```python
from build123d import *

# Parameters (mm, degrees)
F0_R     = 30
F0_R_2   = 17.5
F1_DEPTH = 20
F2_R     = 100
F3_DEPTH = 20.001


with BuildPart() as f1:
    # F0 (on Front) → F1 (new body)
    with BuildSketch(Plane.XZ):
        Circle(F0_R)
        Circle(F0_R_2, mode=Mode.SUBTRACT)
    extrude(amount=-F1_DEPTH)

    # F2 (on face) → F3 (cut, through all)
    with BuildSketch(Plane.XZ):
        Circle(F2_R)
        with BuildLine():
            ThreePointArc((29.9421970705, 1.8614066163), (29.9855457856, 0.9311519438), (30, 0))
            ThreePointArc((30, 0), (25.5026684247, -15.7991741309), (13.3590731187, -26.8614066163))
            Line((13.3590731187, -26.8614066163), (0, -50))
            Line((0, -50), (-13.3590731187, -26.8614066163))
            ThreePointArc((-13.3590731187, -26.8614066163), (-25.9807621135, -15), (-29.9421970705, 1.8614066163))
            Line((-29.9421970705, 1.8614066163), (-43.3012701892, 25))
            Line((-43.3012701892, 25), (-16.5831239518, 25))
            ThreePointArc((-16.5831239518, 25), (0, 30), (16.5831239518, 25))
            Line((16.5831239518, 25), (43.3012701892, 25))
            Line((43.3012701892, 25), (29.9421970705, 1.8614066163))
        make_face(mode=Mode.SUBTRACT)
        with BuildLine():
            Line((-16.5831239518, 25), (16.5831239518, 25))
            ThreePointArc((16.5831239518, 25), (0, 30), (-16.5831239518, 25))
        make_face()
        with BuildLine():
            ThreePointArc((-29.9421970705, 1.8614066163), (-25.9807621135, -15), (-13.3590731187, -26.8614066163))
            Line((-13.3590731187, -26.8614066163), (-29.9421970705, 1.8614066163))
        make_face()
        with BuildLine():
            ThreePointArc((13.3590731187, -26.8614066163), (25.5026684247, -15.7991741309), (30, 0))
            ThreePointArc((30, 0), (29.9855457856, 0.9311519438), (29.9421970705, 1.8614066163))
            Line((29.9421970705, 1.8614066163), (13.3590731187, -26.8614066163))
        make_face()
    extrude(amount=-F3_DEPTH, mode=Mode.SUBTRACT)


solid = f1.part
```
Design review of the part built by this model. Coordinates are the model's own, in mm. Round coordinates to 2 decimals unless told otherwise and drop trailing zeros. Write each loop counter-clockwise with the first axis right and the second up, starting at its lowest first coordinate (ties: lowest second). Pieces come first, ordered by that corner, then holes. Notation, with made-up numbers: (8.25, 35.25) -> (28.25, 35.25) arc R14 cw to (28.25, 43.25) -> close; hole circle Ø3 at (88, 41.5). An arc over 180 degrees is marked (long way). Write item = value, one per line. Start each with the question number.
1) Clearance check with flat-ended pins moving along their axes: pin 1 (12 mm diameter, centred on x = -14.5, z = -5.5, fed in from -Y); pin 2 (6 mm diameter, centred on x = 12.5, y = 15, fed in from -Z); pin 3 (1 mm diameter, centred on y = 5.5, z = -3, fed in from +X); pin 4 (3 mm diameter, centred on x = -3.5, y = 15.5, fed in from -Z). State where each tip first meets the part, or that it passes through.
2) Take a section at B-B, the plane y = 7.75. State the section outline as (x, z) points.
3) Take a section at A-A, the plane x = 0. State the section outline as (y, z) points.
4) Wall thickness on probe 1 along Z at (x, y) = (0, 7.25); probe 2 along X at (y, z) = (14, 16); probe 3 along Z at (x, y) = (-11.5, 13.25): over which ranges is each line inside the solid? List them lowest first. Write a range as from..to.
5) Take a section at C-C, the plane z = 0. State the section outline as (x, y) points, plus the area to 3 significant figures.
6) Mouldability with a two-part tool opening along Z and no side actions: class faces 1 (the face through (-21.535, 9.86, -12.701)), 2 (the face through (0, 10, 25)), 3 (the face through (-13.887, 9.86, -10.648)), 4 (the face through (-7.1, 0, 16.2)) as +Z half, -Z half, draft (parallel to the pull), parting line (faces both ways), or undercut.
7) Take a section at D-D, the plane z = -22.5. State the section outline as (x, y) points, plus the area to 3 significant figures.
Results list:
q1.pin_1 = 0
q1.pin_2 = -28.46
q1.pin_3 = 27.42
q1.pin_4 = -29.93
q2.outline = (-29.94, 1.86) -> (-13.36, -26.86) arc R30 ccw to (13.36, -26.86) -> (29.94, 1.86) arc R30 ccw to (16.58, 25) -> (-16.58, 25) arc R30 ccw to start; hole circle Ø35 at (0, 0)
q3.outline = (0, -30) -> (20, -30) -> (20, -17.5) -> (0, -17.5) -> close; (0, 17.5) -> (20, 17.5) -> (20, 25) -> (0, 25) -> close
q4.probe_1 = -30..-17.5, 17.5..25
q4.probe_2 = -25.38..-7.09, 7.09..25.38
q4.probe_3 = -27.71..-13.19, 13.19..25
q5.outline = (-28.87, 0) -> (-17.5, 0) -> (-17.5, 20) -> (-28.87, 20) -> close; (17.5, 0) -> (28.87, 0) -> (28.87, 20) -> (17.5, 20) -> close
q5.area = 455 mm²
q6.face_1 = -Z half
q6.face_2 = +Z half
q6.face_3 = undercut
q6.face_4 = draft
q7.outline = (-15.88, 0) -> (15.88, 0) -> (15.88, 20) -> (-15.88, 20) -> close
q7.area = 635 mm²
